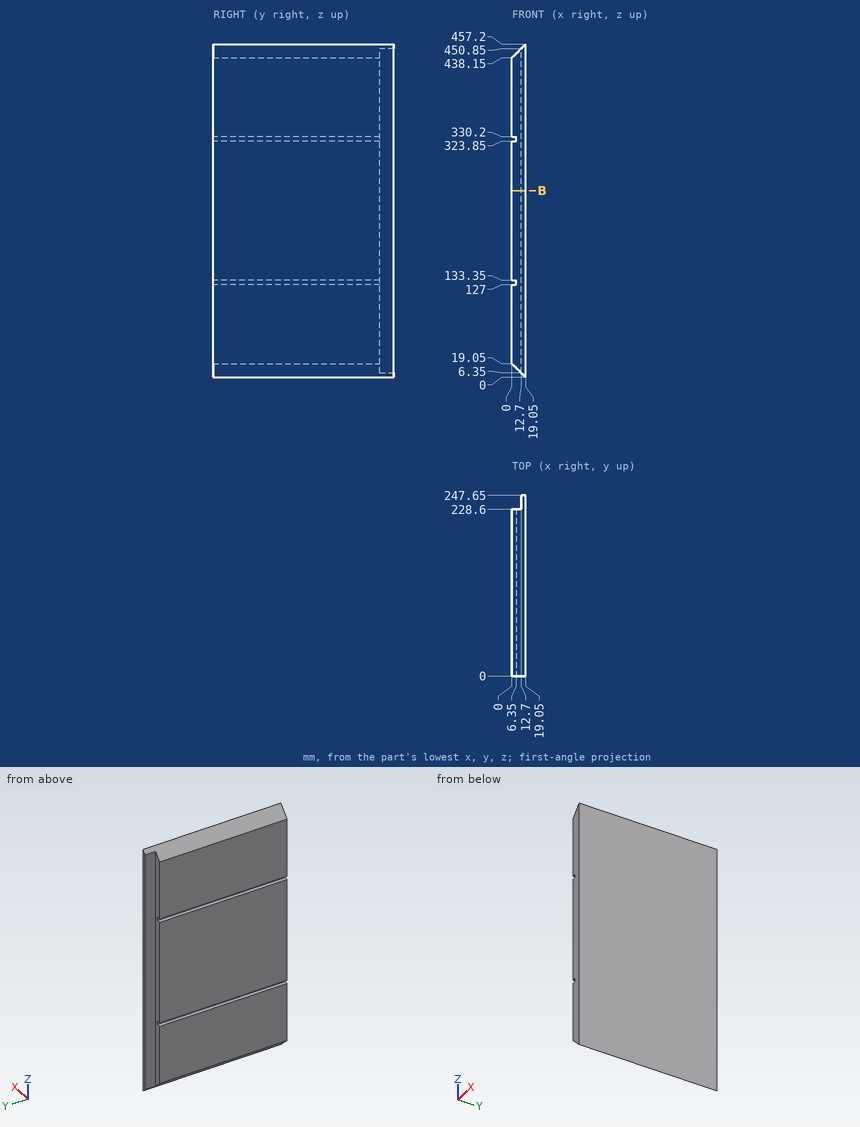
Input: dimensioned drawing with shaded views. Units: mm. Origin: part minimum x, y, z. Give positions to 0.01 mm unless a question says otherwise; leave off trailing zeros. Write each loop counter-clockwise with the first axis right and the second up, starting at its lowest first coordinate (ties: lowest second). Pieces come first, ordered by that corner, then holes. Notation, with made-up numbers: (37.25, -13) -> (82.25, -13) arc R14 cw to (82.25, 4) -> close; hole circle Ø5 at (1, -36). An arc over 180 degrees is marked (long way). Return JSON: item names as keys, results as strings. Group by question number.
1. Pin query (flat end, axial travel): pin 1 Ø3 at (x, y) = (3, 135.5) entering from -Z; pin 2 Ø5 at (x, y) = (2.5, 77) entering from +Z; pin 3 Ø3 at (y, z) = (59.5, 129.5) entering from -X. Return the tip coordinate at first contact, or that it passes through.
2. Material intervals for line 1 (Z direction, x = 6, y = 199); line 2 (Z direction, x = 5, y = 140); line 3 (Y direction, x = 2.25, z = 423), sorted ascending. Write a range as from..to.
3. Section B-B, the plane z = 256. Output: boundary loops of the cut face in (x, y), then the cut area to 3 significant figures.
Determined:
{
 "1": {"pin 1": "stops at z = 14.55", "pin 2": "stops at z = 443.15", "pin 3": "stops at x = 6.35"},
 "2": {"line 1": "z = 13.05..127, 133.35..323.85, 330.2..444.15", "line 2": "z = 14.05..127, 133.35..323.85, 330.2..443.15", "line 3": "y = 0..228.6"},
 "3": {"outline": "(0, 0) -> (19.05, 0) -> (19.05, 247.65) -> (12.7, 247.65) -> (12.7, 228.6) -> (0, 228.6) -> close", "area": "4,480 mm2"}
}
